Could you check a few things on this model? Use its own coordinates, in mm. Give positions to 0.01 mm unless a question says otherwise; leave off trailing zeros. Write each loop counter-clockwise with the first axis right and the second up, starting at its lowest first coordinate (ties: lowest second). Pieces come first, ordered by that corner, then holes. Notation, with made-up numbers: M -7.5,11.25 L 29.5,11.25 A24 ccw 29.5,34.25 Z; hole C 63,67.5 d11. An arc over 180 degrees is marked long. Write each question's results on one line, items separated by ' | '. Start each with the question number.
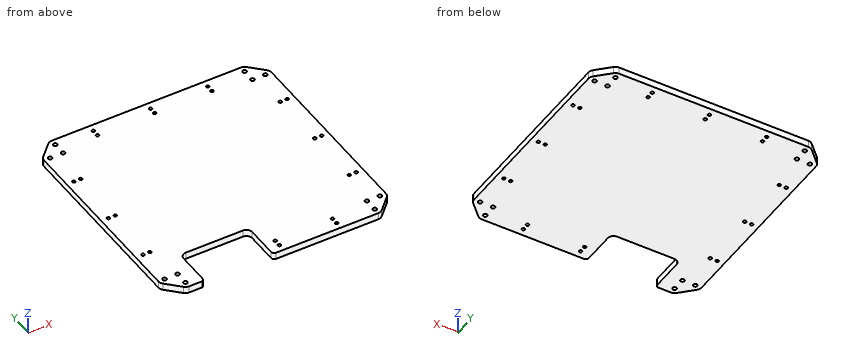
Solid Edge part; units mm, degrees
sketch "Sketch1" plane through (0, 0, 0) normal (0, 0, 1) x (1, 0, 0)
  line L0 (55.1284, -44.4558) -> (55.1284, -375.5442)
  arc A0 (55.1284, -375.5442) -> (58.2624, -383.1102) centre (65.8284, -375.5442) ccw
  line L1 (58.2624, -383.1102) -> (80.8898, -405.7376)
  arc A1 (80.8898, -405.7376) -> (88.4558, -408.8716) centre (88.4558, -398.1716) ccw
  line L2 (88.4558, -408.8716) -> (419.5442, -408.8716)
  arc A2 (419.5442, -408.8716) -> (427.1102, -405.7376) centre (419.5442, -398.1716) ccw
  line L3 (427.1102, -405.7376) -> (449.7376, -383.1102)
  arc A3 (449.7376, -383.1102) -> (452.8716, -375.5442) centre (442.1716, -375.5442) ccw
  line L4 (452.8716, -375.5442) -> (452.8716, -44.4558)
  arc A4 (452.8716, -44.4558) -> (449.7376, -36.8898) centre (442.1716, -44.4558) ccw
  line L5 (449.7376, -36.8898) -> (427.1102, -14.2624)
  arc A5 (427.1102, -14.2624) -> (419.5442, -11.1284) centre (419.5442, -21.8284) ccw
  line L6 (419.5442, -11.1284) -> (88.4558, -11.1284)
  arc A6 (88.4558, -11.1284) -> (80.8898, -14.2624) centre (88.4558, -21.8284) ccw
  line L7 (80.8898, -14.2624) -> (58.2624, -36.8898)
  arc A7 (58.2624, -36.8898) -> (55.1284, -44.4558) centre (65.8284, -44.4558) ccw
  circle A8 centre (65.8284, -44.4558) radius 3.5
  circle A9 centre (88.4558, -44.4558) radius 3.5
  circle A10 centre (88.4558, -21.8284) radius 3.5
  circle A11 centre (419.5442, -21.8284) radius 3.5
  circle A12 centre (419.5442, -44.4558) radius 3.5
  circle A13 centre (442.1716, -44.4558) radius 3.5
  circle A14 centre (419.5442, -398.1716) radius 3.5
  circle A15 centre (442.1716, -375.5442) radius 3.5
  circle A16 centre (88.4558, -398.1716) radius 3.5
  circle A17 centre (88.4558, -375.5442) radius 3.5
  circle A18 centre (65.8284, -375.5442) radius 3.5
  circle A19 centre (419.5442, -375.5442) radius 3.5
extrude "Protrusion1" add sketch "Sketch1" along normal blind 12
sketch "Sketch2" plane through (240, -196, 12) normal (0, 0, 1) x (0, -1, 0)
  circle A0 centre (114, 188.3716) radius 2.7
  circle A1 centre (-86, 200.3716) radius 2.7
  circle A2 centre (-86, 188.3716) radius 2.7
  circle A3 centre (200.3716, 14) radius 2.7
  circle A4 centre (188.3716, 14) radius 2.7
  circle A5 centre (200.3716, -86) radius 2.7
  circle A6 centre (188.3716, -86) radius 2.7
  circle A7 centre (200.3716, 114) radius 2.7
  circle A8 centre (188.3716, 114) radius 2.7
  circle A9 centre (14, -172.3716) radius 2.7
  circle A10 centre (14, -160.3716) radius 2.7
  circle A11 centre (-86, -172.3716) radius 2.7
  circle A12 centre (-86, -160.3716) radius 2.7
  circle A13 centre (114, -172.3716) radius 2.7
  circle A14 centre (114, -160.3716) radius 2.7
  circle A15 centre (-172.3716, 14) radius 2.7
  circle A16 centre (-160.3716, 14) radius 2.7
  circle A17 centre (-172.3716, 114) radius 2.7
  circle A18 centre (-160.3716, 114) radius 2.7
  circle A19 centre (14, 200.3716) radius 2.7
  circle A20 centre (14, 188.3716) radius 2.7
  circle A21 centre (-172.3716, -86) radius 2.7
  circle A22 centre (-160.3716, -86) radius 2.7
  circle A23 centre (114, 200.3716) radius 2.7
extrude "Cutout1" cut sketch "Sketch2" against normal through all
sketch "Sketch3" plane through (254, -210, 12) normal (0, 0, 1) x (1, 0, 0)
  line L0 (-138.8716, -198.8716) -> (-138.8716, -128.8716)
  line L1 (-138.8716, -128.8716) -> (-18.8716, -128.8716)
  line L2 (-18.8716, -128.8716) -> (-18.8716, -198.8716)
extrude "Cutout2" cut sketch "Sketch3" against normal through all material side at (115.1784, -373.8716, 12)
fillet "Round_1" radius 10 2 edges at (115.1284, -338.8716, 6) (235.1284, -338.8716, 6)
fillet "Round_2" radius 5 2 edges at (115.1284, -408.8716, 6) (235.1284, -408.8716, 6)
properties material "Wood, Ash"
Q1. If we section it at B-B (x = 163): Please give me the cut outline in (y, z).
Q2. I'm going to push a flat-ended pin straight in: P1, Ø5, axis at x = 159.5, z = 9, coming from the -Y side. Where does the tip first touch, or does it pass through?
Q3. Please list where these lines run through material, in increasing order: line 1 (X direction, y = -110, z = 3.5); line 2 (Y direction, x = 254, z = 9.5); line 3 (X direction, y = -359.5, z = 9.25). Write a range as [from, to].
Q4. If we section it at A-A (z = 9.5): Count the separate pieces of the cut face and the enclosed holes in it, plus the area to 3 significant figures.
Determined:
1) outline: M -338.87,0 L -11.13,0 L -11.13,12 L -338.87,12 Z
2) P1: stops at y = -338.87
3) line 1: x = [55.13, 64.93], [70.33, 76.93], [82.33, 425.67], [431.07, 437.67], [443.07, 452.87] | line 2: y = [-408.87, -399.07], [-393.67, -387.07], [-381.67, -38.33], [-32.93, -26.33], [-20.93, -11.13] | line 3: x = [55.13, 115.13], [235.13, 452.87]
4) separate pieces: 1 | enclosed holes: 34 | area: 147,000 mm²
